Build history of the part. All positions in model axes, mm. Face numbers are marked on the shaded views. Give positions to 0.01 mm unless a question says otherwise; leave off trailing zeros. Write each loop counter-clockwise with the first axis right and the second up, starting at its lowest first coordinate (ties: lowest second). Pieces come first, ordered by that corner, then holes.
from build123d import *

# Parameters (mm, degrees)
CYLINDER003_R     = 5.25
CYLINDER003_DEPTH = 6
CYLINDER002_R     = 15
CYLINDER002_DEPTH = 6
BOX_W             = 30
BOX_H             = 6
BOX_DEPTH         = 37
FILLET001_R       = 25
BOX001_W          = 30
BOX001_H          = 16
BOX001_DEPTH      = 37
CYLINDER_R        = 11
CYLINDER_DEPTH    = 25
CYLINDER001_R     = 16
CYLINDER001_DEPTH = 25
FILLET_R          = 2


with BuildPart() as cilindro003:
    # Cylinder003 → Cylinder003 (new body)
    with BuildSketch(Plane(origin=(27, 3, 38), x_dir=(1, 0, 0), z_dir=(0, -1, 0))):
        Circle(CYLINDER003_R)
    extrude(amount=CYLINDER003_DEPTH)


with BuildPart() as cilindro002:
    # Cylinder002 → Cylinder002 (new body)
    with BuildSketch(Plane(origin=(27, 3, 38), x_dir=(1, 0, 0), z_dir=(0, -1, 0))):
        Circle(CYLINDER002_R)
    extrude(amount=CYLINDER002_DEPTH)


with BuildPart() as fillet001:
    # Box → Box (new body)
    with BuildSketch(Plane(origin=(12, -3, 0), x_dir=(1, 0, 0), z_dir=(0, 0, 1))):
        with Locations((15, 3)):
            Rectangle(BOX_W, BOX_H)
    extrude(amount=BOX_DEPTH)

    # Fusion: union Cilindro002
    add(cilindro002.part)

    # Cut001: cut Cilindro003
    add(cilindro003.part, mode=Mode.SUBTRACT)

    # Fillet001
    fillet001_edges = [fillet001.edges().sort_by_distance(p)[0] for p in [
        (42, 0, 0),
    ]]
    fillet(fillet001_edges, radius=FILLET001_R)


with BuildPart() as cubo001:
    # Box001 → Box001 (new body)
    with BuildSketch(Plane(origin=(-24, -8, 0), x_dir=(1, 0, 0), z_dir=(0, 0, 1))):
        with Locations((15, 8)):
            Rectangle(BOX001_W, BOX001_H)
    extrude(amount=BOX001_DEPTH)


with BuildPart() as cilindro:
    # Cylinder → Cylinder (new body)
    with BuildSketch(Plane.XY):
        Circle(CYLINDER_R)
    extrude(amount=CYLINDER_DEPTH)


with BuildPart() as fusion001:
    # Cylinder001 → Cylinder001 (new body)
    with BuildSketch(Plane.XY):
        Circle(CYLINDER001_R)
    extrude(amount=CYLINDER001_DEPTH)

    # Cut: cut Cilindro
    add(cilindro.part, mode=Mode.SUBTRACT)

    # Cut002: cut Cubo001
    add(cubo001.part, mode=Mode.SUBTRACT)

    # Fillet
    fillet_edges = [fusion001.edges().sort_by_distance(p)[0] for p in [
        (-13.856406, -8, 12.5),
        (-13.856406, 8, 12.5),
    ]]
    fillet(fillet_edges, radius=FILLET_R)

    # Fusion001: union Fillet001
    add(fillet001.part)


solid = fusion001.part
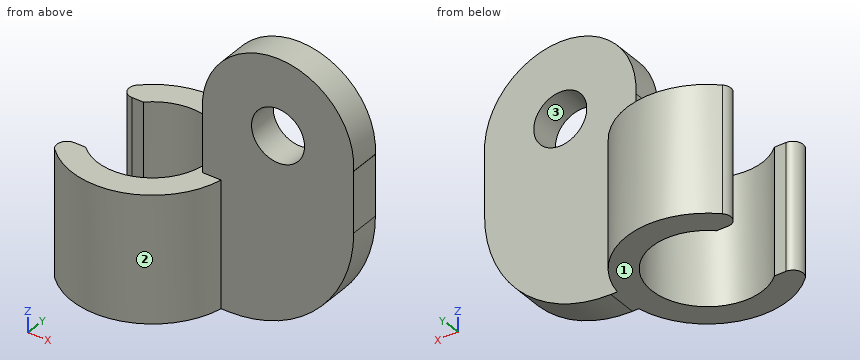
(1) Saw through at D-D, the plane z = 19. List the corners of the cut face in (x, y).
(2) Mould opens along Z. For the marked faces 1, 2 and 3 say: +Z half, -Z half, draft (parallel to the pull), parting line (faces both ways), or undercut.
(3) Saw through at A-A, the plane x = 0. List the corners of the cut face in (y, z), plus the area to 3 significant figures.
(4) Probe line 1 (Y direction, x = -0.5, z = 21.5); line 2 (Y direction, x = 30.5, z = 24); line 3 (Y direction, x = -3, z = 21.5). List the from-to ranges inside material, lowest first.
(5) Drop flat-ended pins along their axis: pin 1 (1 mm diameter, centred on x = 13, z = 40.5, fed in from +Y); pin 2 (13.5 mm diameter, centred on x = 27, z = 38, fed in from -Y); pin 3 (6.5 mm diameter, centred on y = 1, z = 33, fed in from -X). Give the stop position or say it passes through.
(6) Saw through at C-C, the plane z = 38. List the corners of the cut face in (x, y).
Computed values:
1. outline: (-11.2, -11.43) arc R16 ccw to (15.72, -3) - (41.27, -3) - (41.27, 3) - (15.72, 3) arc R16 ccw to (-11.2, 11.43) arc R2 ccw to (-9.8, 8) - (-7.55, 8) arc R11 cw (long way) to (-7.55, -8) - (-9.8, -8) arc R2 ccw to start
2. face 1: -Z half
2. face 2: draft
2. face 3: undercut
3. outline: (-16, 0) - (-11, 0) - (-11, 25) - (-16, 25) - close; (11, 0) - (16, 0) - (16, 25) - (11, 25) - close
3. area: 250 mm2
4. line 1: y = -15.99 to -10.99, 10.99 to 15.99
4. line 2: y = -3 to 3
4. line 3: y = -15.72 to -10.58, 10.58 to 15.72
5. pin 1: stops at y = 3
5. pin 2: stops at y = -3
5. pin 3: stops at x = 12
6. outline: (12, -3) - (21.75, -3) - (21.75, 3) - (12, 3) - close; (32.25, -3) - (42, -3) - (42, 3) - (32.25, 3) - close
